Input: part model. Units: mm. Frame: model coordinates. Face numbers are marked on the shaded views. Give positions to 0.01 mm unless a question says otherwise; leave off trailing zeros. Loops run counter-clockwise (first coordinate to the right, second up) from the corner with the lowest first, then second, coordinate; pieces in that order, holes last. Notation, with made-up numbers: (-37, -16) -> (-25, -16) arc R16 ccw to (-25, 2) -> close; hole circle Ø9 at (47, 46.25). An arc over 180 degrees is marked (long way). Answer as a JSON object with one key per item and string values.
Autodesk Inventor part; units mm, degrees
ref_plane "Work Plane1" through (-12, 0, -11) normal (0, 0, 1) x (1, 0, 0)
ref_plane "YZ Plane" through (0, 0, 0) normal (1, 0, 0) x (0, 1, 0)
ref_plane "XZ Plane" through (0, 0, 0) normal (0, 1, 0) x (-1, 0, 0)
ref_plane "Work Plane1" through (-12, 0, -11) normal (0, 0, 1) x (1, 0, 0)
sketch "Boceto6" plane through (0, 0, 0) normal (0, 1, 0) x (-1, 0, 0)
  circle A0 centre (9.21, 17.5305) radius 6
  circle A1 centre (9.21, 17.5305) radius 8
  arc A2 (0.5354, 26.5305) -> (17.8847, 26.5305) centre (9.21, 17.5305) ccw
  circle A3 centre (9.21, 7.5305) radius 1.5
  line L0 (9.21, 17.5305) -> (9.21, 26.5305)
  line L1 (9.21, 26.5305) -> (17.8847, 26.5305)
  line L2 (17.8847, 26.5305) -> (0.5354, 26.5305)
  point P0 (0, 0)
  dimension "d143" = 12
  dimension "d144" = 16
  dimension "d145" = 25
  dimension "d146" = 3
  dimension "d147" = 10
  dimension "d148" = 9
extrude "Extrusión11" add sketch "Boceto6" along normal blind 12 contours A1
extrude "Extrusión12" add sketch "Boceto6" against normal blind 2 contours A1 | L1 A2 L2
properties part number "Buje de Soporte de Motor" material "Acetal Resin, White"
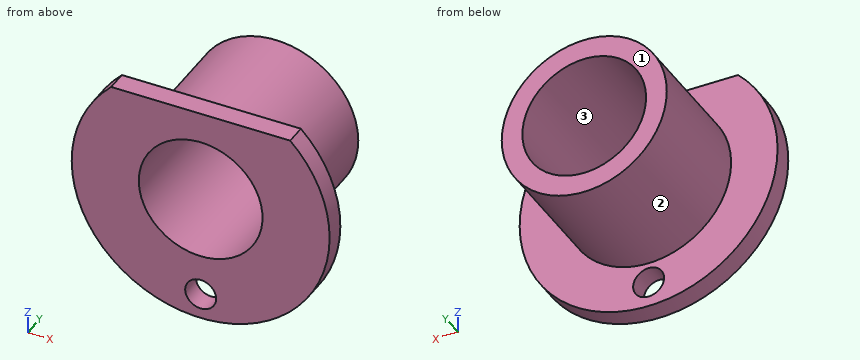
Q1. Ray query, line 1 along Z through (x, y) = (-9.21, -0.85); line 2 along Z through (x, y) = (-9.21, 2.5); line 3 along Y through (x, z) = (-7.75, 8). Return the intervals inside material, ascending.
Evaluation:
{"line 1": "z = 5.03 to 6.03, 9.03 to 11.53, 23.53 to 26.53", "line 2": "z = 9.53 to 11.53, 23.53 to 25.53", "line 3": "y = -2 to 0"}
Q2. Section A-A, the plane x = -9.21. Return the cut outline in (y, z).
Evaluation:
{"outline": "(-2, 5.03) -> (0, 5.03) -> (0, 6.03) -> (-2, 6.03) -> close; (-2, 9.03) -> (0, 9.03) -> (0, 9.53) -> (12, 9.53) -> (12, 11.53) -> (-2, 11.53) -> close; (-2, 23.53) -> (12, 23.53) -> (12, 25.53) -> (0, 25.53) -> (0, 26.53) -> (-2, 26.53) -> close"}
Q3. Draft query along Z for the marked faces 1, 2 and 3. Return one class per face: +Z half, -Z half, draft (parallel to the pull), parting line (faces both ways), or undercut.
Evaluation:
{"face 1": "draft", "face 2": "parting line", "face 3": "undercut"}
Q4. Section C-C, the plane z = 12. Return the cut outline in (x, y), then the cut area to 3 significant figures.
Evaluation:
{"outline": "(-20.42, -2) -> (-11.54, -2) -> (-11.54, 12) -> (-14.99, 12) -> (-14.99, 0) -> (-20.42, 0) -> close; (-6.88, -2) -> (2, -2) -> (2, 0) -> (-3.43, 0) -> (-3.43, 12) -> (-6.88, 12) -> close", "area": "118 mm2"}
Q5. Section D-D, the plane y = -0.5. Return the cut outline in (x, z), then the cut area to 3 significant figures.
Evaluation:
{"outline": "(-17.88, 26.53) arc R12.5 ccw (long way) to (-0.54, 26.53) -> close; hole circle Ø12 at (-9.21, 17.53); hole circle Ø3 at (-9.21, 7.53)", "area": "329 mm2"}
Q6. Pin query (flat end, axial travel): pin 1 (5 mm diameter, centred on x = -9.21, z = 7.53, fed in from +Y); pin 2 (2 mm diameter, centred on x = -5, y = 3.5, fed in from +Z); pin 3 (3 mm diameter, centred on y = 8, z = 12, fed in from +X); pin 4 (5 mm diameter, centred on y = 10, z = 17, fed in from +X). Return the tip coordinate at first contact, or that it passes through.
Evaluation:
{"pin 1": "stops at y = 12", "pin 2": "stops at z = 24.86", "pin 3": "stops at x = -2.3", "pin 4": "stops at x = -1.21"}
Q7. Section B-B, the plane x = -14. Return the cut outline in (y, z).
Evaluation:
{"outline": "(-2, 5.98) -> (0, 5.98) -> (0, 11.12) -> (12, 11.12) -> (12, 13.92) -> (-2, 13.92) -> close; (-2, 21.14) -> (12, 21.14) -> (12, 23.94) -> (0, 23.94) -> (0, 26.53) -> (-2, 26.53) -> close"}
